from build123d import *

# Parameters (mm, degrees)
BOSS_EXTRUDE1_DEPTH = 10
FILLET1_R           = 2
FILLET2_R           = 2
FILLET3_R           = 2
FILLET4_R           = 2
SKETCH2_W           = 11.181044811
SKETCH2_H           = 7.229971792
CUT_EXTRUDE1_DEPTH  = 4


with BuildPart() as part:
    # Sketch1 → Boss-Extrude1 (new body)
    with BuildSketch(Plane.XY):
        Polygon((14, 0), (0, 0), (0, 25), (5, 25), (5, 5), (14, 5), align=None)
    extrude(amount=BOSS_EXTRUDE1_DEPTH)

    # Fillet1
    fillet1_edges = [part.edges().sort_by_distance(p)[0] for p in [
        (2.5, 25, 10),
    ]]
    fillet(fillet1_edges, radius=FILLET1_R)

    # Fillet2
    fillet2_edges = [part.edges().sort_by_distance(p)[0] for p in [
        (2.5, 25, 0),
    ]]
    fillet(fillet2_edges, radius=FILLET2_R)

    # Fillet3
    fillet3_edges = [part.edges().sort_by_distance(p)[0] for p in [
        (14, 2.5, 10),
    ]]
    fillet(fillet3_edges, radius=FILLET3_R)

    # Fillet4
    fillet4_edges = [part.edges().sort_by_distance(p)[0] for p in [
        (14, 2.5, 0),
    ]]
    fillet(fillet4_edges, radius=FILLET4_R)

    # Sketch2 → Cut-Extrude1 (cut)
    with BuildSketch(Plane.XZ):
        with Locations((6.674906448, 5.176903909)):
            Rectangle(SKETCH2_W, SKETCH2_H)
    extrude(amount=-CUT_EXTRUDE1_DEPTH, mode=Mode.SUBTRACT)


solid = part.part
Input: part model. Units: mm. Frame: model coordinates. A direction names the side the tool comes from. Round coordinates to 2 decimals unless told otherwise and drop trailing zeros. Order: outer loops, then holes, each group sorted by start corner. A loop starts at its lowest first (then second) coordinate and runs counter-clockwise, first axis right, second up. Notation, with made-up numbers: (89, -16.75) - (105, -16.75) arc R22 ccw to (105, -10.75) - close; hole circle Ø8 at (21.25, -19.5). An arc over 180 degrees is marked (long way). Use a Markdown table: item, result.
1. Section D-D on y = 9.75. Return the cut outline in (x, z).
Evaluation:
| item | result |
|---|---|
| outline | (0, 0) - (5, 0) - (5, 10) - (0, 10) - close |
2. Section A-A on y = 3.75. Return the cut outline in (x, z).
Evaluation:
| item | result |
|---|---|
| outline | (0, 0) - (12, 0) arc R2 ccw to (14, 2) - (14, 8) arc R2 ccw to (12, 10) - (0, 10) - close; hole (1.08, 1.56) - (12.27, 1.56) - (12.27, 8.79) - (1.08, 8.79) - close |
3. First-contact query: pin 1 (6 mm diameter, centred on x = 12, z = 7, fed in from +Y); pin 2 (2 mm diameter, centred on x = 4.5, z = 7, fed in from -Y); pin 3 (2 mm diameter, centred on y = 17, z = 3.5, fed in from +X). Flat tips, straight axial feed; report the tip coordinate or a pass-through.
Evaluation:
| item | result |
|---|---|
| pin 1 | y = 5 |
| pin 2 | y = 4 |
| pin 3 | x = 5 |
4. Access query for faces 4 (the face through (3, 9, 10)), 5 (the face through (5, 15, 5)), 6 (the face through (7, 2, 8.792)). Directions: +Z, -Z, +X, -X, +Y, -Y. A direction counts if a zero-diameter tool reaches every point of the face in a straight line with its end or side. Return the directions, or none.
Evaluation:
| item | result |
|---|---|
| face 4 | +Z, +X, -X, +Y, -Y |
| face 5 | +Z, -Z, +X, +Y |
| face 6 | -Y |
5. Mould query, pull axis Z, two halves, no side actions, for faces 1 (the face through (9, 5, 5)), 2 (the face through (12.265, 2, 5)), 3 (the face through (13.4, 2.46, 9.43)). Classes: +Z half, -Z half, draft (parallel to the pull), parting line (faces both ways), or undercut.
Evaluation:
| item | result |
|---|---|
| face 1 | draft |
| face 2 | undercut |
| face 3 | +Z half |
6. Section B-B on z = 4.5. Return the cut outline in (x, y).
Evaluation:
| item | result |
|---|---|
| outline | (0, 0) - (1.08, 0) - (1.08, 4) - (12.27, 4) - (12.27, 0) - (14, 0) - (14, 5) - (5, 5) - (5, 25) - (0, 25) - close |
7. Section C-C on x = 2.5. Return the cut outline in (y, z).
Evaluation:
| item | result |
|---|---|
| outline | (0, 0) - (23, 0) arc R2 ccw to (25, 2) - (25, 8) arc R2 ccw to (23, 10) - (0, 10) - (0, 8.79) - (4, 8.79) - (4, 1.56) - (0, 1.56) - close |
8. Material intervals for probe 1 along X at (y, z) = (1.5, 3); probe 2 along Z at (x, y) = (11.25, 2); probe 3 along X at (y, z) = (8.5, 8), sorted ascending.
Evaluation:
| item | result |
|---|---|
| probe 1 | 0 to 1.08, 12.27 to 14 |
| probe 2 | 0 to 1.56, 8.79 to 10 |
| probe 3 | 0 to 5 |
